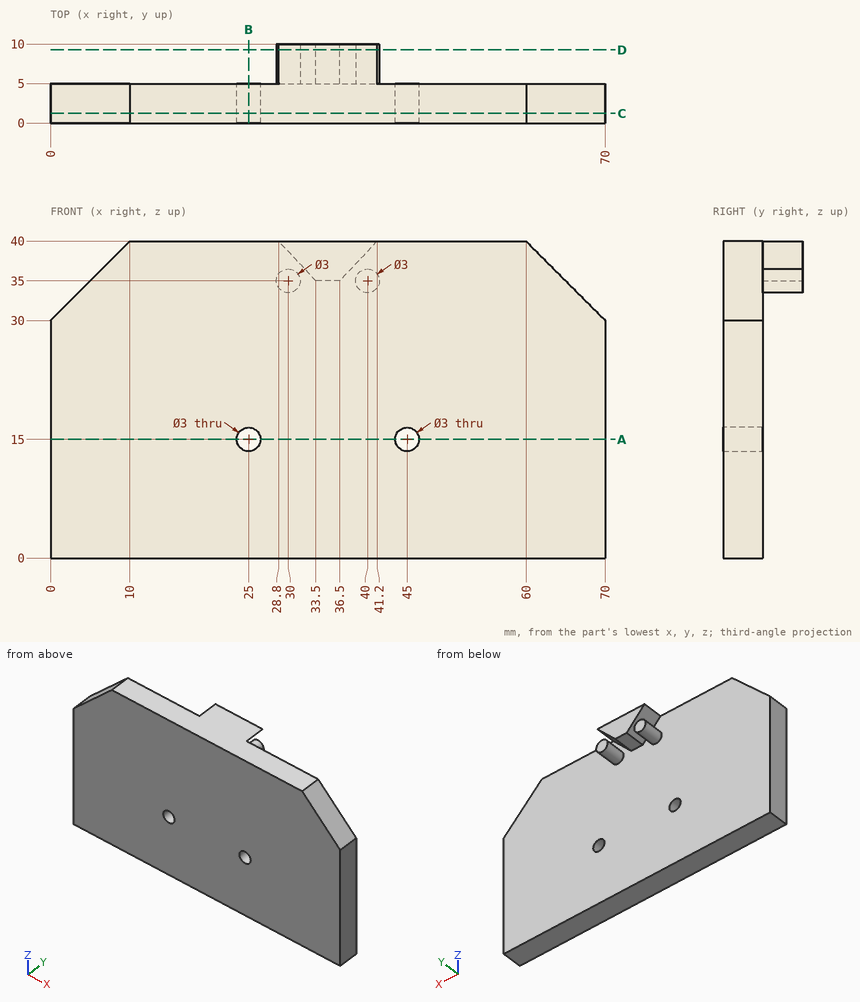
Can you work these out from the drawing? Everything is in mm from the part's minimum corner. Coordinates: 2 decimals unless noted, no trailing zeros. Write each loop counter-clockwise with the first axis right and the second up, starting at its lowest first coordinate (ties: lowest second). Pieces come first, ordered by that corner, then holes. Notation, with made-up numbers: (-5, -31.75) -> (11, -31.75) arc R26 cw to (11, -3.75) -> close; hole circle Ø9 at (-38.75, 1). An arc over 180 degrees is marked (long way). Write each question's results on one line, items separated by ' | '. Start each with the question number.
Q1. Imagine slicing it at B-B (x = 25). Write out the boundary of the cut face in (y, z).
Q2. Imagine slicing it at D-D (y = 9.25). Write out the boundary of the cut face in (x, z).
Q3. Imagine slicing it at C-C (y = 1.25). Write out the boundary of the cut face in (x, z), then the cut area to 3 significant figures.
Q4. I'm going to push flat-ended pins straight in: pin 1 (2.5 mm diameter, centred on x = 25, z = 15, fed in from -Y); pin 2 (12 mm diameter, centred on x = 30, z = 17.5, fed in from +Y); pin 3 (1.5 mm diameter, centred on x = 35, y = 7.5, fed in from -Z); pin 4 (3 mm diameter, centred on y = 5.5, z = 32, fed in from -X). Where does each tip first touch, or does it pass through?
Q5. If I drill on probe 1 along X at (y, z) = (3.5, 15); probe 2 along Y at (x, z) = (60, 13); probe 3 along Z at (x, y) = (66.5, 2.75), over which ranges is the centre line in solid material (lowest first)?
Q6. Imagine slicing it at A-A (z = 15). Write out the boundary of the cut face in (x, y).
Taken from the geometry:
1) outline: (0, 0) -> (5, 0) -> (5, 13.5) -> (0, 13.5) -> close; (0, 16.5) -> (5, 16.5) -> (5, 40) -> (0, 40) -> close
2) outline: circle Ø3 at (30, 35); (28.8, 40) -> (33.5, 35) -> (36.5, 35) -> (41.2, 40) -> close; circle Ø3 at (40, 35)
3) outline: (0, 0) -> (70, 0) -> (70, 30) -> (60, 40) -> (10, 40) -> (0, 30) -> close; hole circle Ø3 at (25, 15); hole circle Ø3 at (45, 15) | area: 2,690 mm^2
4) pin 1: passes through | pin 2: stops at y = 5 | pin 3: stops at z = 35 | pin 4: stops at x = 0.59
5) probe 1: x = 0 to 23.5, 26.5 to 43.5, 46.5 to 70 | probe 2: y = 0 to 5 | probe 3: z = 0 to 33.5
6) outline: (0, 0) -> (23.5, 0) -> (23.5, 5) -> (0, 5) -> close; (26.5, 0) -> (43.5, 0) -> (43.5, 5) -> (26.5, 5) -> close; (46.5, 0) -> (70, 0) -> (70, 5) -> (46.5, 5) -> close
